Input: dimensioned drawing with shaded views. Units: mm. Origin: part minimum x, y, z. Round coordinates to 2 decimals unless told otherwise and drop trailing zeros. Loops run counter-clockwise (first coordinate to the right, second up) from the corner with the lowest first, then second, coordinate; pieces in that order, holes last. Notation, with made-up numbers: M 28,67.5 L 76,67.5 A22 cw 76,87.5 Z; hole C 18.25,43.5 d8. An arc over 180 degrees is marked long. Answer as a JSON object with one key per item and string values.
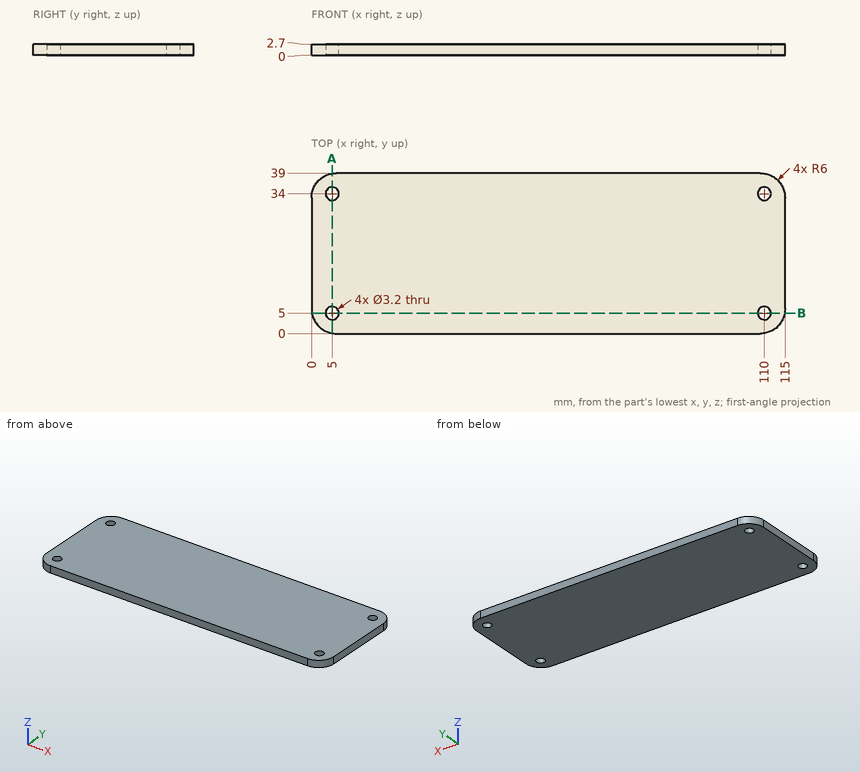
Item 1: Section A-A on x = 5. Return the cut outline in (y, z).
Answer sheet:
{"outline": "M 0.08,0 L 3.4,0 L 3.4,2.7 L 0.08,2.7 Z; M 6.6,0 L 32.4,0 L 32.4,2.7 L 6.6,2.7 Z; M 35.6,0 L 38.92,0 L 38.92,2.7 L 35.6,2.7 Z"}
Item 2: Line query: probe 1 along X at (y, z) = (4, 1.95); probe 2 along Y at (x, z) = (110, 1.4); probe 3 along X at (y, z) = (6, 2.2). Output: solid intervals per line, ascending. Write a range as from..to.
Answer sheet:
{"probe 1": "x = 0.34..3.75, 6.25..108.75, 111.25..114.66", "probe 2": "y = 0.08..3.4, 6.6..32.4, 35.6..38.92", "probe 3": "x = 0..3.75, 6.25..108.75, 111.25..115"}
Item 3: Contact query for a flat-ended pin moving along its axis: pin 1 Ø2.5 at (x, y) = (110, 34) entering from -Z. Output: stop coordinate, or through.
Answer sheet:
{"pin 1": "passes through"}
Item 4: Section B-B on y = 5. Return the cut outline in (x, z).
Answer sheet:
{"outline": "M 0.08,0 L 3.4,0 L 3.4,2.7 L 0.08,2.7 Z; M 6.6,0 L 108.4,0 L 108.4,2.7 L 6.6,2.7 Z; M 111.6,0 L 114.92,0 L 114.92,2.7 L 111.6,2.7 Z"}
